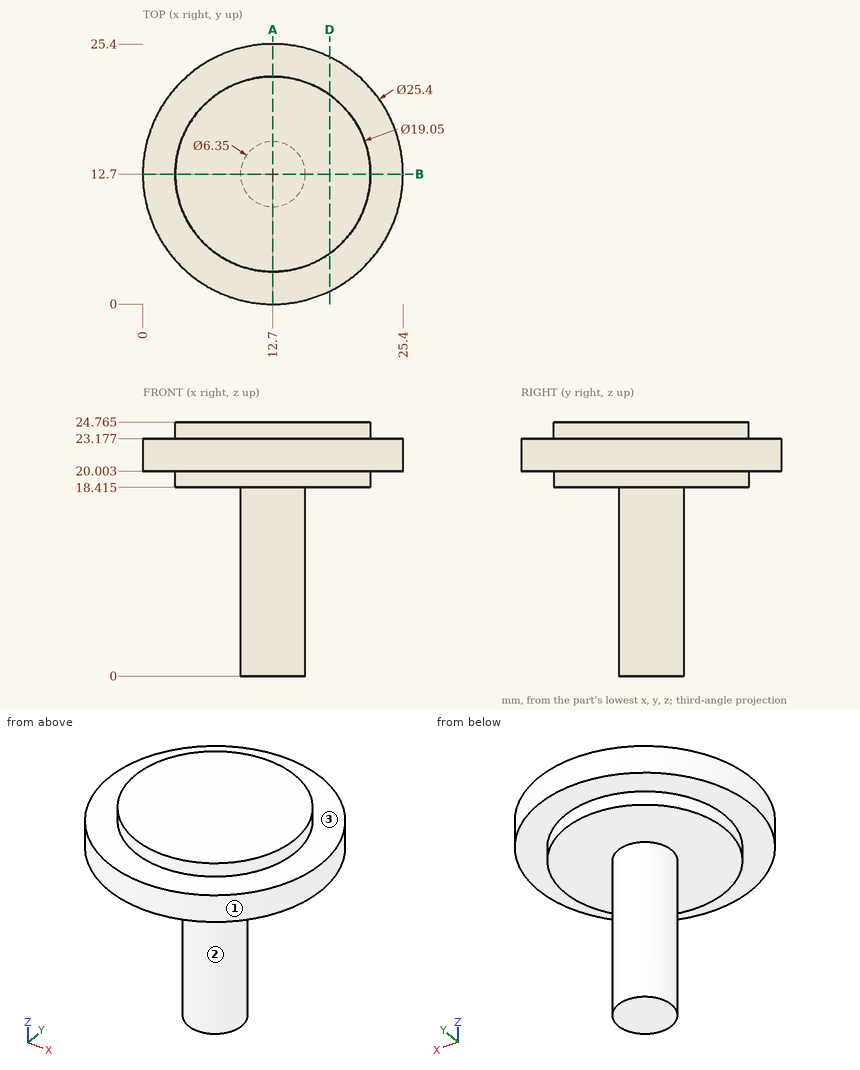
Check sheet for the drawn part. Datum: minimum x, y, z corner. Units: mm. A direction names the side the tool comes from. Round coordinates to 2 decimals unless told otherwise and drop trailing zeros. Write each loop counter-clockwise with the first axis right and the second up, starting at its lowest first coordinate (ties: lowest second). Pieces come first, ordered by that corner, then holes. Notation, with made-up numbers: (31, 73.5) - (84, 73.5) arc R24 ccw to (84, 92.5) - close; hole circle Ø4 at (61.5, 33). An arc over 180 degrees is marked (long way). Return JSON: item names as keys, results as strings.
Q1. Depth check by flat-ended pin: P1, Ø6, axis at x = 22.5, y = 9, coming from the +Z side (1 decimal); P2, Ø5, axis at y = 7.5, z = 9, coming from the +X side; P3, Ø6, axis at x = 14.5, y = 4, coming from the -Z side (1 decimal); P4, Ø5, axis at y = 11, z = 3, coming from the -X side (1 decimal). Enter the tip coordinate at first touch or a pass-through.
Returned:
{"P1": "stops at z = 24.8", "P2": "stops at x = 14.37", "P3": "stops at z = 18.4", "P4": "stops at x = 9.5"}
Q2. Cross-section at A-A (x = 12.7). Record the boundary of the cut face in (y, z) (1 decimal).
Returned:
{"outline": "(0, 20) - (3.2, 20) - (3.2, 18.4) - (9.5, 18.4) - (9.5, 0) - (15.9, 0) - (15.9, 18.4) - (22.2, 18.4) - (22.2, 20) - (25.4, 20) - (25.4, 23.2) - (22.2, 23.2) - (22.2, 24.8) - (3.2, 24.8) - (3.2, 23.2) - (0, 23.2) - close"}
Q3. Cross-section at D-D (x = 18.25). Record the boundary of the cut face in (y, z) (1 decimal), then the cut area to 3 significant figures.
Returned:
{"outline": "(1.3, 20) - (5, 20) - (5, 18.4) - (20.4, 18.4) - (20.4, 20) - (24.1, 20) - (24.1, 23.2) - (20.4, 23.2) - (20.4, 24.8) - (5, 24.8) - (5, 23.2) - (1.3, 23.2) - close", "area": "122 mm²"}
Q4. Scan lines: L1, parallel to Z at x = 1.5, y = 7.5; L2, parallel to Z at x = 13.75, y = 5 (1 decimal); L3, parallel to Y at x = 12.5, z = 5. Record each from-to range of solid material in increasing order. Write a range as from..to.
Returned:
{"L1": "z = 20..23.18", "L2": "z = 18.4..24.8", "L3": "y = 9.53..15.87"}
Q5. Access from +Z, -Z, +X, -X, +Y, -Y to the whole of each face (thin tool, end or side, straight path). Record for the marked faces 1, 2 and 3.
Returned:
{"face 1": "+Z, -Z", "face 2": "-Z", "face 3": "+Z"}
